The listing builds one solid part. Answer for the finished solid, in the listing's coordinates (mm). Give positions to 0.01 mm unless a question says otherwise; leave off trailing zeros. Order: outer loops, then holes, each group sorted by start corner. A loop starts at its lowest first (then second) coordinate and runs counter-clockwise, first axis right, second up.
```python
from build123d import *

# Parameters (mm, degrees)
SKIZZE2_R                       = 1.23
AUFSATZ_LINEAR_AUSTRAGEN1_DEPTH = 6
FASE1_SIZE                      = 0.27
FASE1_SIZE2                     = 0.155884573
FASE2_SIZE                      = 0.27
FASE2_SIZE2                     = 0.155884573


with BuildPart() as part:
    # Skizze2 → Aufsatz-Linear austragen1 (new, symmetric)
    with BuildSketch(Plane(origin=(0, 0, 0), x_dir=(1, 0, 0), z_dir=(0, 1, 0))):
        Polygon((3.175426481, 0), (1.58771324, 2.75), (-1.58771324, 2.75), (-3.175426481, 0), (-1.58771324, -2.75), (1.58771324, -2.75), align=None)
        with Locations(Location((0, 0, 0), (0, 0, 270))):
            Circle(SKIZZE2_R, mode=Mode.SUBTRACT)
    extrude(amount=AUFSATZ_LINEAR_AUSTRAGEN1_DEPTH, both=True)

    # Fase1
    fase1_edges = [part.edges().sort_by_distance(p)[0] for p in [
        (0, 6, -1.23),
    ]]
    fase1_side = [part.faces().sort_by_distance(p)[0] for p in [
        (2.308811699, 6, -1.332993056),
    ]]
    chamfer(fase1_edges, length=FASE1_SIZE, length2=FASE1_SIZE2, reference=fase1_side[0])

    # Fase2
    fase2_edges = [part.edges().sort_by_distance(p)[0] for p in [
        (0, -6, -1.23),
    ]]
    fase2_side = [part.faces().sort_by_distance(p)[0] for p in [
        (2.308811699, -6, -1.332993056),
    ]]
    chamfer(fase2_edges, length=FASE2_SIZE, length2=FASE2_SIZE2, reference=fase2_side[0])

    # Skizze3 → Schnitt-Rotation1 (revolve, cut)
    with BuildSketch(Plane.XY, mode=Mode.PRIVATE) as schnitt_rotation1_sk:
        Polygon((-2.3, 6), (-4.116867346, 6), (-4.116867346, 4.951031149), align=None)
        Polygon((-2.3, -6), (-4.116867346, -6), (-4.116867346, -4.951031149), align=None)
    revolve(schnitt_rotation1_sk.sketch.rotate(Axis((0, 5.844115427, 0), (0, -1, 0)), 119.99999992), axis=Axis((0, 5.844115427, 0), (0, -1, 0)), mode=Mode.SUBTRACT)


solid = part.part
```
1) Straight lines are drawn through the part: probe 1 along Z at (x, y) = (0.5, 2); probe 2 along X at (y, z) = (1, -0.2); probe 3 along Z at (x, y) = (-1, 4.75). For each, find the intervals that lie inside material, in ascending order.
Geometry says:
probe 1: z = -2.75 to -1.12, 1.12 to 2.75
probe 2: x = -3.06 to -1.21, 1.21 to 3.06
probe 3: z = -2.75 to -0.72, 0.72 to 2.75
2) Given P1, Ø1, axis at y = -1.5, z = 2, coming from the -X side, flat-ended and moving along its own axis, determine where the tip first touches the part or whether it passes through.
Geometry says:
P1: stops at x = -2.31
3) Find section B-B (x = 0). Write down the section's boundary in (y, z).
Geometry says:
outline: (-6, -2.3) - (-5.74, -2.75) - (5.74, -2.75) - (6, -2.3) - (6, -1.5) - (5.84, -1.23) - (-5.84, -1.23) - (-6, -1.5) - close; (-6, 1.5) - (-5.84, 1.23) - (5.84, 1.23) - (6, 1.5) - (6, 2.3) - (5.74, 2.75) - (-5.74, 2.75) - (-6, 2.3) - close
4) Find section A-A (y = -2). Write down the section's boundary in (x, z).
Geometry says:
outline: (-3.18, 0) - (-1.59, -2.75) - (1.59, -2.75) - (3.18, 0) - (1.59, 2.75) - (-1.59, 2.75) - close; hole circle Ø2.46 at (0, 0)
5) For a pull along Z with two mould halves and no side action, classify faces 1 (the cylindrical face through (1.04, -0.08, 0.66)), 2 (the flat face through (0, 0, 2.75)), 3 (the flat face through (2, -6, 0)) as +Z half, -Z half, draft (parallel to the pull), parting line (faces both ways), or undercut.
Geometry says:
face 1: undercut
face 2: +Z half
face 3: draft
